Geometry check sheet. Reference: drawing and pictorial views, mm from the part's lowest x, y, z. A direction names the side the tool comes from. Round coordinates to 2 decimals unless told otherwise and drop trailing zeros. Order: outer loops, then holes, each group sorted by start corner. A loop starts at its lowest first (then second) coordinate and runs counter-clockwise, first axis right, second up.
(1) Sectioned sample at A-A, the plane z = 19.05. Enter the section's corners in (x, y), and give its area (3 significant figures).
(2) Depth check by flat-ended pin: pin 1 (4 mm diameter, centred on x = 101, z = 23.5, fed in from -Y); pin 2 (6 mm diameter, centred on x = 35.5, z = 18, fed in from -Y); pin 3 (3 mm diameter, centred on x = 80.5, z = 16, fed in from -Y); pin 4 (5 mm diameter, centred on x = 101, z = 12, fed in from -Y). Enter the tip coordinate at first touch or a pass-through.
(3) Sectioned sample at C-C, the plane x = 68. Enter the section's corners in (y, z), and give its area (3 significant figures).
(4) Sectioned sample at D-D, the plane z = 29. Enter the section's corners in (x, y) (1 decimal).
(5) Thickness scan on probe 1 along Y at (x, z) = (81, 20.5) (1 decimal); probe 2 along Y at (x, z) = (52.5, 15.5); probe 3 along Z at (x, y) = (62, 22.5) (1 decimal). Record the ranges inside material, lowest first.
(6) Sectioned sample at B-B, the plane y = 21.5. Enter the section's corners in (x, z).
(7) Mould release check, pull along Z, two halves, no side actions. Record for the marked faces 1, 2 and 3: released by +Z, released by -Z, zero draft, split by the parting line, or undercut.
(8) Tool access check on the marked faces 4 and 5. Record the directions out of +Z, -Z, +X, -X, +Y, -Y that give a thin tool (end or side, any length) a straight path to the whole face; none if there is none.
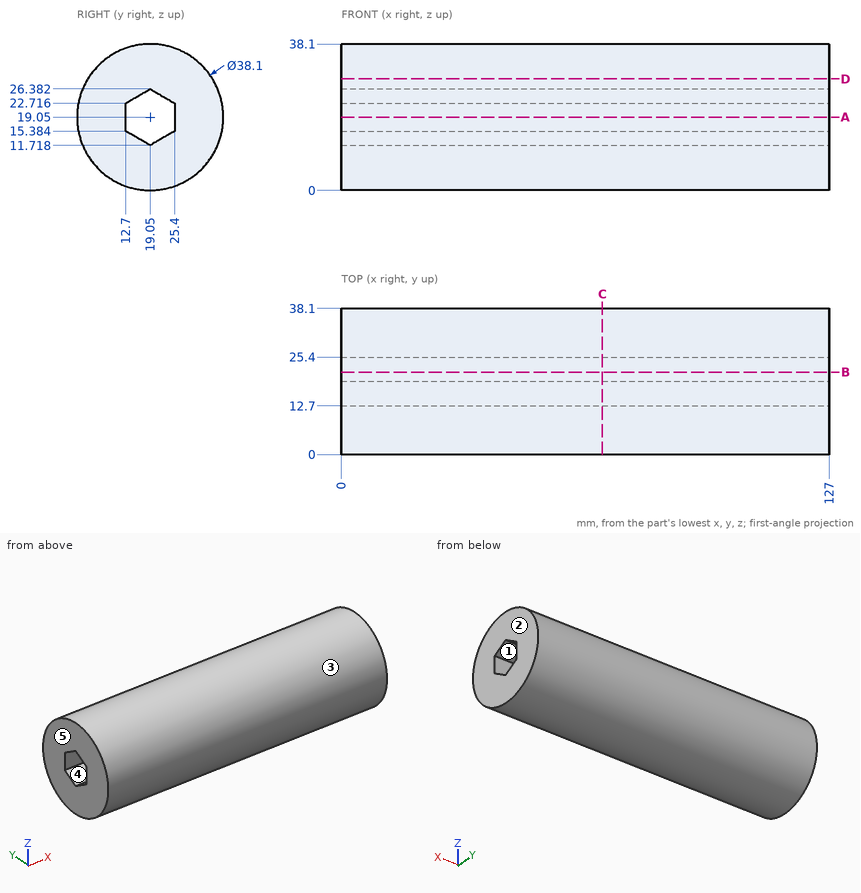
Derived:
1. outline: (0, 0) - (127, 0) - (127, 12.7) - (0, 12.7) - close; (0, 25.4) - (127, 25.4) - (127, 38.1) - (0, 38.1) - close
1. area: 3,230 mm2
2. pin 1: stops at y = 0.16
2. pin 2: stops at y = 0
2. pin 3: stops at y = 0.06
2. pin 4: stops at y = 0.55
3. outline: circle Ø38.1 at (19.05, 19.05); hole (12.7, 15.38) - (19.05, 11.72) - (25.4, 15.38) - (25.4, 22.72) - (19.05, 26.38) - (12.7, 22.72) - close
3. area: 1,000 mm2
4. outline: (0, 2.8) - (127, 2.8) - (127, 35.3) - (0, 35.3) - close
5. probe 1: y = 0.1 to 12.7, 25.4 to 38
5. probe 2: y = 0.33 to 12.7, 25.4 to 37.77
5. probe 3: z = 0.3 to 13.7, 24.4 to 37.8
6. outline: (0, 0.16) - (127, 0.16) - (127, 13.13) - (0, 13.13) - close; (0, 24.97) - (127, 24.97) - (127, 37.94) - (0, 37.94) - close
7. face 1: undercut
7. face 2: zero draft
7. face 3: split by the parting line
8. face 4: +X, -X
8. face 5: +Z, -Z, -X, +Y, -Y
